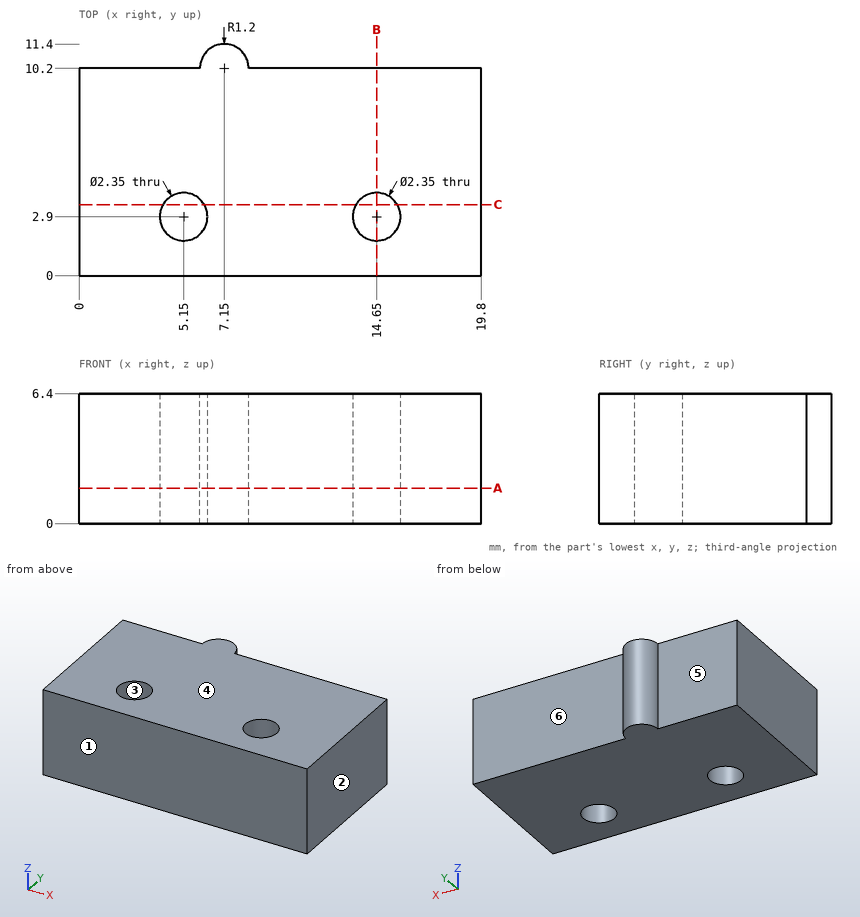
For this review, use the dimensioned drawing (mm, ordinates from the lowest corner) and the shaded views. A direction names the side the tool comes from. Give positions to 0.01 mm unless a question says otherwise; leave off trailing zeros. Loops run counter-clockwise (first coordinate to the right, second up) from the corner with the lowest first, then second, coordinate; pieces in that order, holes last. Notation, with made-up numbers: (-28, 60.5) -> (28, 60.5) arc R24 cw to (28, 84.5) -> close; hole circle Ø10 at (13.25, -24). An arc over 180 degrees is marked (long way). One line per question, with ' | ' between items. Start each with the question number.
(1) Insertion check: P1, Ø3, axis at x = 14.65, y = 2.9, coming from the +Z side; P2, Ø2, axis at x = 2.5, z = 5, coming from the +Y side. Each pin has a flat end and moves straight along its axis. Give the tip position at first contact, or say it passes through.
(2) Draft analysis for pull direction X (two halves, no side actions). For the marked faces 1, 2 and 3, state which applies: +X half, -X half, draft (parallel to the pull), parting line (faces both ways), or undercut.
(3) We need section C-C (y = 3.5). State the section outline as (x, z) points.
(4) We need section A-A (z = 1.75). State the section outline as (x, y) points (3 decimals), and give its area (3 significant figures).
(5) For the marked faces 4, 5 and 6, list the 3-axis set-ups (+Z, -Z, +X, -X, +Y, -Y) from which the entire face can be reached by the end or side of a thin tool; tool diameter is ignored.
(6) For line 1 (Y direction, x = 5.15, z = 5.25) (3 decimals); line 2 (X direction, y = 2.5, z = 6.25); line 3 (Y direction, x = 10.5, z = 3), list the stretches that pass through material, from the lowest coordinate up.
(7) We need section B-B (x = 14.65). State the section outline as (y, z) points (3 decimals).
The answers:
1) P1: stops at z = 6.4 | P2: stops at y = 10.2
2) face 1: draft | face 2: +X half | face 3: undercut
3) outline: (0, 0) -> (4.14, 0) -> (4.14, 6.4) -> (0, 6.4) -> close; (6.16, 0) -> (13.64, 0) -> (13.64, 6.4) -> (6.16, 6.4) -> close; (15.66, 0) -> (19.8, 0) -> (19.8, 6.4) -> (15.66, 6.4) -> close
4) outline: (0, 0) -> (19.8, 0) -> (19.8, 10.2) -> (8.35, 10.2) arc R1.2 ccw to (5.95, 10.2) -> (0, 10.2) -> close; hole circle Ø2.35 at (5.15, 2.9); hole circle Ø2.35 at (14.65, 2.9) | area: 196 mm^2
5) face 4: +Z, +X, -X, +Y, -Y | face 5: +Z, -Z, -X, +Y | face 6: +Z, -Z, +X, +Y
6) line 1: y = 0 to 1.725, 4.075 to 10.2 | line 2: x = 0 to 4.05, 6.25 to 13.55, 15.75 to 19.8 | line 3: y = 0 to 10.2
7) outline: (0, 0) -> (1.725, 0) -> (1.725, 6.4) -> (0, 6.4) -> close; (4.075, 0) -> (10.2, 0) -> (10.2, 6.4) -> (4.075, 6.4) -> close
